Part model, mm, in its own coordinate system. Coordinates: 2 decimals unless noted, no trailing zeros. Order: outer loops, then holes, each group sorted by start corner. A loop starts at its lowest first (then second) coordinate and runs counter-clockwise, first axis right, second up.
1) Wall check: L1, parallel to X at y = -9.8, z = 412.5; L2, parallel to X at y = 0, z = 412.5. Give the ranges that are in metal, low to high.
2) Cut at A-A (z = 351). List the corners of the cut face in (x, y).
3) Pin check, flat tip, straight feed: pin 1 Ø5 at (x, z) = (-5, 63.5) entering from +Y. Stop position of the tip, or through.
4) Cut at B-B (y = 0.75). List the corners of the cut face in (x, z).
```python
from build123d import *

# Parameters (mm, degrees)
SKETCH_1_W          = 20
SKETCH_1_H          = 20
SKETCH_1_W_2        = 19
SKETCH_1_H_2        = 19
EXTRUDE_1_DEPTH     = 498
SKETCH_2_R          = 2
CUT_EXTRUDE_1_DEPTH = 20


with BuildPart() as part:
    # 草图1 → 凸台-拉伸1 (new body)
    with BuildSketch(Plane.XY):
        Rectangle(SKETCH_1_W, SKETCH_1_H)
        Rectangle(SKETCH_1_W_2, SKETCH_1_H_2, mode=Mode.SUBTRACT)
    extrude(amount=EXTRUDE_1_DEPTH)

    # 草图2 → 切除-拉伸1 (cut)
    with BuildSketch(Plane(origin=(0, 10, 0), x_dir=(1, 0, 0), z_dir=(0, 1, 0))):
        with Locations(Location((-5, -12.5, 0), (0, 0, 270))):
            Circle(SKETCH_2_R)
        with Locations(Location((-5, -34.5, 0), (0, 0, 270))):
            Circle(SKETCH_2_R)
        with Locations(Location((-5, -85.5, 0), (0, 0, 270))):
            Circle(SKETCH_2_R)
        with Locations(Location((-5, -63.5, 0), (0, 0, 270))):
            Circle(SKETCH_2_R)
        with Locations(Location((-5, -434.5, 0), (0, 0, 270))):
            Circle(SKETCH_2_R)
        with Locations(Location((-5, -412.5, 0), (0, 0, 270))):
            Circle(SKETCH_2_R)
        with Locations(Location((-5, -463.5, 0), (0, 0, 270))):
            Circle(SKETCH_2_R)
        with Locations(Location((-5, -485.5, 0), (0, 0, 270))):
            Circle(SKETCH_2_R)
        with Locations(Location((5, -485.5, 0), (0, 0, 270))):
            Circle(SKETCH_2_R)
        with Locations(Location((5, -463.5, 0), (0, 0, 270))):
            Circle(SKETCH_2_R)
        with Locations(Location((5, -434.5, 0), (0, 0, 270))):
            Circle(SKETCH_2_R)
        with Locations(Location((5, -412.5, 0), (0, 0, 270))):
            Circle(SKETCH_2_R)
        with Locations(Location((5, -85.5, 0), (0, 0, 270))):
            Circle(SKETCH_2_R)
        with Locations(Location((5, -63.5, 0), (0, 0, 270))):
            Circle(SKETCH_2_R)
        with Locations(Location((5, -34.5, 0), (0, 0, 270))):
            Circle(SKETCH_2_R)
        with Locations(Location((5, -12.5, 0), (0, 0, 270))):
            Circle(SKETCH_2_R)
    extrude(amount=-CUT_EXTRUDE_1_DEPTH, mode=Mode.SUBTRACT)


solid = part.part
```
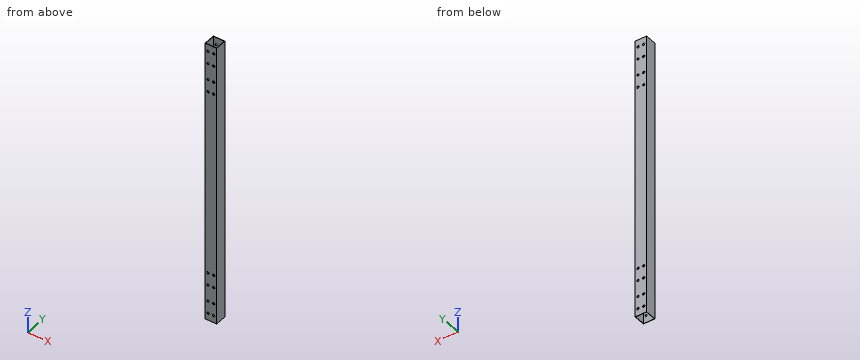
Geometry check:
1. L1: x = -10 to -7, -3 to 3, 7 to 10
1. L2: x = -10 to -9.5, 9.5 to 10
2. outline: (-10, -10) - (10, -10) - (10, 10) - (-10, 10) - close; hole (-9.5, -9.5) - (9.5, -9.5) - (9.5, 9.5) - (-9.5, 9.5) - close
3. pin 1: stops at y = 10
4. outline: (-10, 0) - (-9.5, 0) - (-9.5, 498) - (-10, 498) - close; (9.5, 0) - (10, 0) - (10, 498) - (9.5, 498) - close
